from build123d import *

# Parameters (mm, degrees)
F1_DEPTH      = 25
F1_DEPTH_BACK = 25
F2_DEPTH      = 25
F2_DEPTH_BACK = 25
F3_T1_DEPTH   = 55.8032253547
F4_START      = 24
F4_DEPTH      = 1


# Not quite as in the source:
# - a fillet or chamfer that OpenCascade refuses, or shapes differently, is made with other operations: its cross-section is extruded or revolved along the edge and cut away or added


with BuildPart() as f1:
    # F0 (on Right) → F1 (new body, two sides)
    with BuildSketch(Plane.YZ) as f1_sk:
        with BuildLine():
            ThreePointArc((-0.474586405, -1.4229433383), (-0.9510831171, -1.1599314222), (-1.3023647132, -0.7442084075))
            Line((-1.3023647132, -0.7442084075), (-19.8057450128, -11.3175685788))
            ThreePointArc((-19.8057450128, -11.3175685788), (-21.1992188281, -12.2788787263), (-22.4105694786, -13.461467444))
            ThreePointArc((-22.4105694786, -13.461467444), (-24.7010613056, -21.6868174799), (-19.8057450128, -28.6824314212))
            Line((-19.8057450128, -28.6824314212), (0, -40))
            Line((0, -40), (0, -38.8482488931))
            Line((0, -38.8482488931), (-19.3096060745, -27.8141882791))
            ThreePointArc((-19.3096060745, -27.8141882791), (-23.8443556293, -20), (-19.3096060745, -12.1858117209))
            Line((-19.3096060745, -12.1858117209), (-0.474586405, -1.4229433383))
        make_face()
        with BuildLine():
            Line((0, 0), (-1.3023647132, -0.7442084075))
            ThreePointArc((-1.3023647132, -0.7442084075), (-0.9510831171, -1.1599314222), (-0.474586405, -1.4229433383))
            Line((-0.474586405, -1.4229433383), (0, -1.1517511069))
            Line((0, -1.1517511069), (0, 0))
        make_face()
    extrude(amount=F1_DEPTH)
    extrude(f1_sk.sketch, amount=-F1_DEPTH_BACK)

    # F0 (on Right) → F2 (join, two sides)
    with BuildSketch(Plane.YZ) as f2_sk:
        Polygon((3, -40.5625346074), (0, -38.8482488931), (0, -40), (3, -41.7142857143), align=None)
    extrude(amount=F2_DEPTH)
    extrude(f2_sk.sketch, amount=-F2_DEPTH_BACK)

    # F3: fillet of radius 2 on 1 edges, made by hand

    # F3_s2 → F3_t1 (cut)
    with BuildSketch(Plane.YZ.offset(-27.9016126774)):
        with BuildLine():
            ThreePointArc((1.9922778767, -39.9866933941), (2.7298201862, -40.7193260419), (3, -41.7231796783))
            Line((3, -41.7231796783), (3, -40.5625346074))
            Line((3, -40.5625346074), (1.9922778767, -39.9866933941))
        make_face()
    extrude(amount=F3_T1_DEPTH, mode=Mode.SUBTRACT)

    # F0 (on Right) → F4 (join)
    with BuildSketch(Plane.YZ.offset(F4_START)):
        with BuildLine():
            Line((0, -38.8482488931), (0, -1.5))
            ThreePointArc((0, -1.5), (-0.2404006993, -1.4806105172), (-0.474586405, -1.4229433383))
            Line((-0.474586405, -1.4229433383), (-19.3096060745, -12.1858117209))
            ThreePointArc((-19.3096060745, -12.1858117209), (-23.8443556293, -20), (-19.3096060745, -27.8141882791))
            Line((-19.3096060745, -27.8141882791), (0, -38.8482488931))
        make_face()
        with BuildLine():
            ThreePointArc((-0.474586405, -1.4229433383), (-0.2404006993, -1.4806105172), (0, -1.5))
            Line((0, -1.5), (0, -1.1517511069))
            Line((0, -1.1517511069), (-0.474586405, -1.4229433383))
        make_face()
    extrude(amount=F4_DEPTH)


solid = f1.part
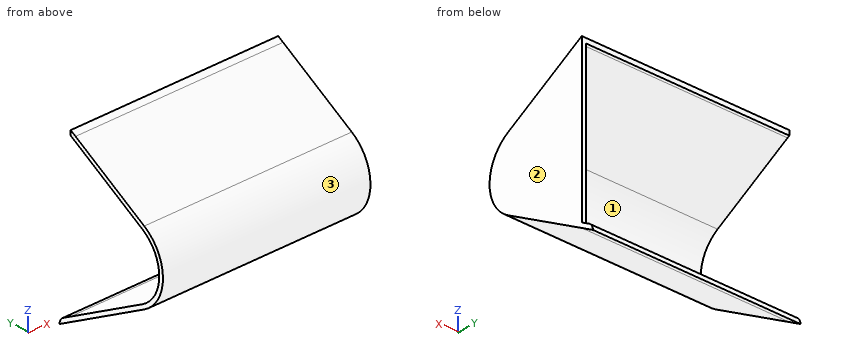
Geometry check sheet. Reference: the model listing, model coordinates, mm. Face numbers are marked on the shaded views. Coordinates: 2 decimals unless noted, no trailing zeros. Order: outer loops, then holes, each group sorted by start corner. A loop starts at its lowest first (then second) coordinate and runs counter-clockwise, first axis right, second up. Notation, with made-up numbers: (70.25, 29.25) - (97.25, 29.25) arc R18 cw to (97.25, 41.25) - close; hole circle Ø5 at (-31, 73). An arc over 180 degrees is marked (long way). Answer in a Markdown table with one row per item. Add a question column.
1) Cross-section at B-B, the plane y = -9.25. Record the cut outline in (x, z).
2) Release check for a two-part mould opening along Z. For the marked faces 1, 2 and 3 record: +Z half, -Z half, draft (parallel to the pull), parting line (faces both ways), or undercut.
3) Material ranges on line 1 along X through (y, z) = (-18, -11.5); line 2 along Z through (x, y) = (-4, -23); line 3 along Z through (x, y) = (18, -4.75), recorded low to high. Write a range as [from, to].
4) Gauge pin test, flat ends, axial feed: P1, Ø12, axis at x = -2.5, z = -11, coming from the -Y side; P2, Ø2, axis at x = 16.5, y = -10, coming from the -Z side; P3, Ø1, axis at x = 4.5, z = -7, coming from the +Y side. Record the tip position at first contact, or that the pin passes through.
5) Cross-section at A-A, the plane x = 1. Record the cut outline in (y, z), then the cut area to 3 significant figures.
6) Cross-section at C-C, the plane z = -18. Record the cut outline in (x, y), then the cut area to 3 significant figures.
7) Cross-section at D-D, the plane y = -14.5. Record the cut outline in (x, z), then the cut area to 3 significant figures.
Check result:
| question | item | result |
|---|---|---|
| 1 | outline | (-25, -34.71) - (25, -34.71) - (25, -5.29) - (-25, -5.29) - (-25, -6.44) - (24, -6.44) - (24, -33.56) - (-25, -33.56) - close |
| 2 | face 1 | undercut |
| 2 | face 2 | draft |
| 2 | face 3 | parting line |
| 3 | line 1 | x = [24, 25] |
| 3 | line 2 | z = [-25.79, -23.81], [-16.19, -14.21] |
| 3 | line 3 | z = [-37.29, -36.13], [-3.87, -2.71] |
| 4 | P1 | stops at y = -24.38 |
| 4 | P2 | stops at z = -34.86 |
| 4 | P3 | stops at y = -9.36 |
| 5 | outline | (-19.81, -28.68) - (3, -41.71) arc R2 ccw to (1.99, -39.99) - (-19.31, -27.81) arc R9 cw to (-19.31, -12.19) - (0, -1.15) - (0, 0) - (-19.81, -11.32) arc R10 ccw to start |
| 5 | area | 68.3 mm² |
| 6 | outline | (-25, -24.64) - (25, -24.64) - (25, 0) - (24, 0) - (24, -23.62) - (-25, -23.62) - close |
| 6 | area | 74.8 mm² |
| 7 | outline | (-25, -31.71) - (25, -31.71) - (25, -8.29) - (-25, -8.29) - (-25, -9.44) - (24, -9.44) - (24, -30.56) - (-25, -30.56) - close |
| 7 | area | 136 mm² |
